Here's the drawing with two shaded views (mm, measured from the low corner). I have some questions. Coordinates: 2 decimals unless noted, no trailing zeros. Write each loop counter-clockwise with the first axis right and the second up, starting at its lowest first coordinate (ties: lowest second). Pieces come first, ordered by that corner, then holes.
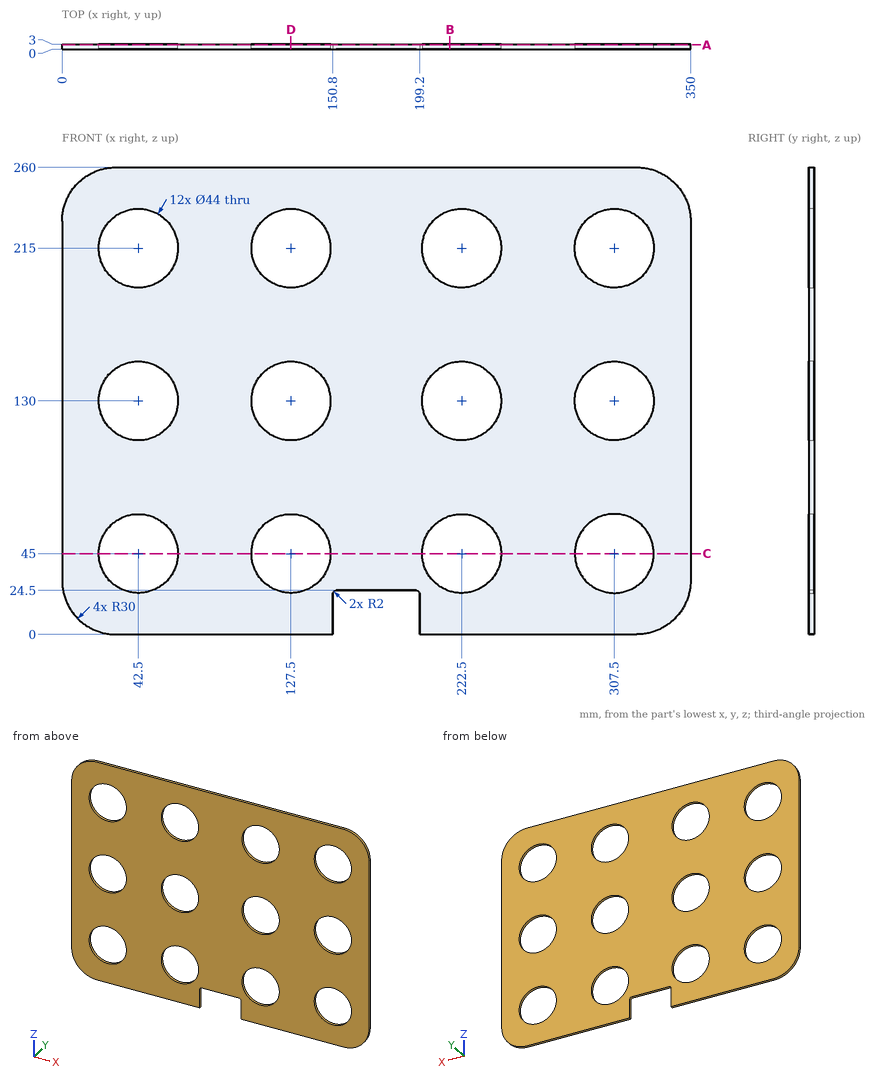
1. Please list where these lines run through material, in increasing order: line 1 along Z through (x, y) = (307.5, 1.85); line 2 along Z through (x, y) = (58.5, 1.9); line 3 along X through (y, z) = (1.5, 195).
Verdict:
line 1: z = 0 to 23, 67 to 108, 152 to 193, 237 to 260
line 2: z = 0 to 29.9, 60.1 to 114.9, 145.1 to 199.9, 230.1 to 260
line 3: x = 0 to 33.33, 51.67 to 118.33, 136.67 to 213.33, 231.67 to 298.33, 316.67 to 350
2. I want a section at D-D on x = 127.5. Please give me the cut outline in (y, z).
Verdict:
outline: (0, 0) - (3, 0) - (3, 23) - (0, 23) - close; (0, 67) - (3, 67) - (3, 108) - (0, 108) - close; (0, 152) - (3, 152) - (3, 193) - (0, 193) - close; (0, 237) - (3, 237) - (3, 260) - (0, 260) - close
3. I want a section at B-B on x = 216. Please give me the cut outline in (y, z).
Verdict:
outline: (0, 0) - (3, 0) - (3, 23.98) - (0, 23.98) - close; (0, 66.02) - (3, 66.02) - (3, 108.98) - (0, 108.98) - close; (0, 151.02) - (3, 151.02) - (3, 193.98) - (0, 193.98) - close; (0, 236.02) - (3, 236.02) - (3, 260) - (0, 260) - close
4. I want a section at A-A on y = 2.55. Give the number of separate pieces and of enclosed holes in the cut face, plus the area to 3 significant figures.
Verdict:
separate pieces: 1
enclosed holes: 12
area: 70,800 mm2
5. I want a section at C-C on z = 45. Please give me the cut outline in (x, y).
Verdict:
outline: (0, 0) - (20.5, 0) - (20.5, 3) - (0, 3) - close; (64.5, 0) - (105.5, 0) - (105.5, 3) - (64.5, 3) - close; (149.5, 0) - (200.5, 0) - (200.5, 3) - (149.5, 3) - close; (244.5, 0) - (285.5, 0) - (285.5, 3) - (244.5, 3) - close; (329.5, 0) - (350, 0) - (350, 3) - (329.5, 3) - close
6. For pin 1 (0.9 mm diameter, centred on y = 2, z = 15, fed in from +X); pin 2 (10 mm diameter, centred on x = 166, z = 176, fed in from -Y), each with a flat end and sliding along its axis, tell me the tip position at first contact or that it passes through.
Verdict:
pin 1: stops at x = 346.24
pin 2: stops at y = 0
